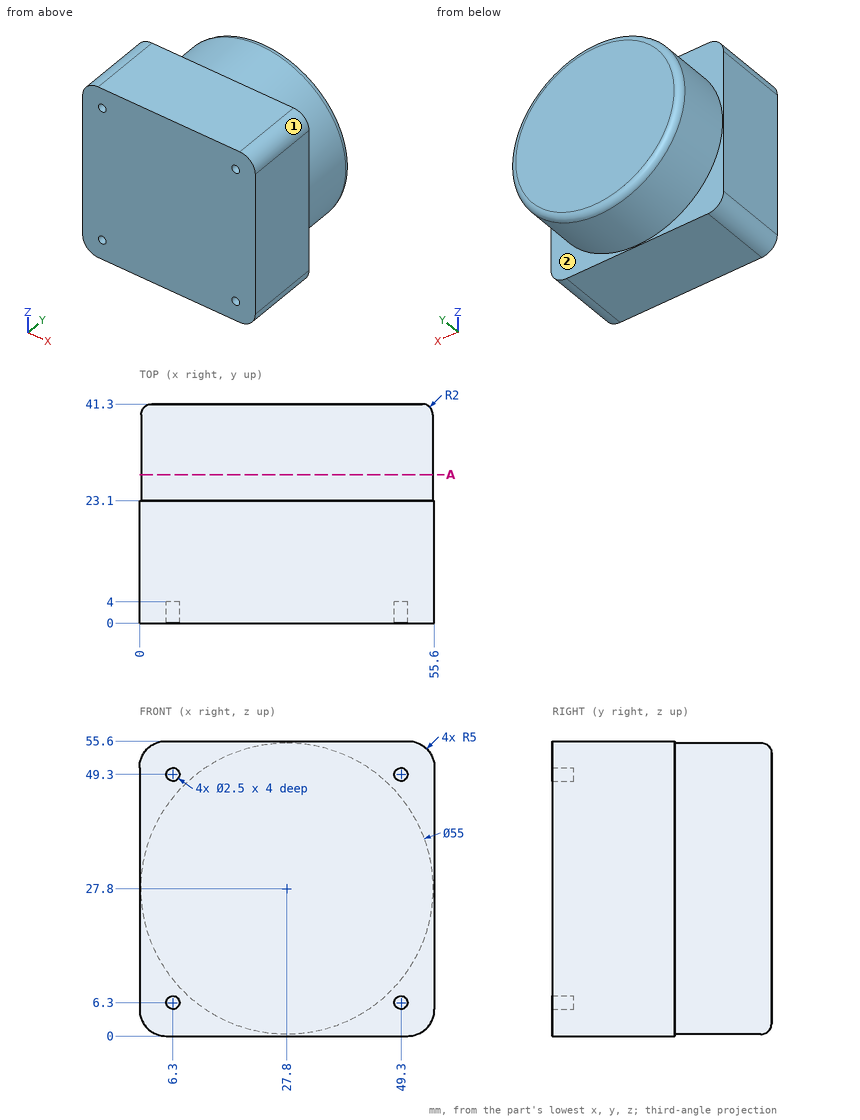
Answer from the drawing. Dimensions are ordinates in mm from the lowest x, y and z of the part. A direction names the side the tool comes from. Round coordinates to 2 decimals unless told otherwise and drop trailing zeros. Write each loop counter-clockwise with the first axis right and the second up, starting at its lowest first coordinate (ties: lowest second). Pieces come first, ordered by that corner, then holes.
1. Given pin 1 Ø3 at (x, z) = (6.3, 49.3) entering from +Y; pin 2 Ø4 at (y, z) = (35.5, 27.5) entering from +X, each flat-ended and moving along its own axis, determine where each tip first touches the part or whether it passes through.
2. Straight lines are drawn through the part: L1, parallel to X at y = 2.25, z = 49.3; L2, parallel to Y at x = 52.5, z = 4.5. For each, find the intervals that lie inside material, in ascending order.
3. Which of the six approach directions +Z, -Z, +X, -X, +Y, -Y give full straight-line access (tool end or side, diameter ignored) to the marked faces 1 and 2?
4. The part is cut by section A-A, the plane y = 28. Determine the outline of the cut face in (x, z), then the cut area to 3 significant figures.
Values:
1. pin 1: stops at y = 23.1
1. pin 2: stops at x = 55.3
2. L1: x = 0 to 5.05, 7.55 to 48.05, 50.55 to 55.6
2. L2: y = 0 to 23.1
3. face 1: +Z, +X, +Y, -Y
3. face 2: +Y
4. outline: circle Ø55 at (27.8, 27.8)
4. area: 2,380 mm2
